Work out the finished part from the listing and answer in its coordinate system (mm). Coordinates: 2 decimals unless noted, no trailing zeros. Order: outer loops, then holes, each group sorted by start corner. A loop starts at its lowest first (then second) coordinate and runs counter-clockwise, first axis right, second up.
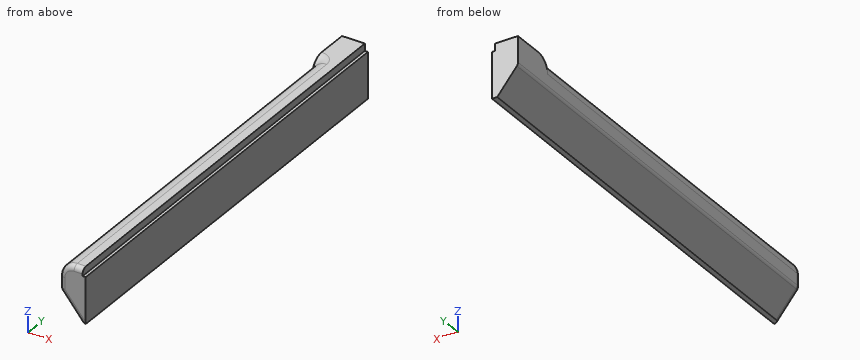
```python
from build123d import *

# Parameters (mm, degrees)
F1_DEPTH = 430
F3_W     = 14
F3_H     = 3.9684094482
F5_DEPTH = 385.0010001
F6_R     = 5


with BuildPart() as f1:
    # F0 (on Front) → F1 (new body)
    with BuildSketch(Plane.XZ):
        with BuildLine():
            Line((-3.0895532303, -0.0301503569), (-25.4895532303, -0.0301503569))
            Line((-25.4895532303, -0.0301503569), (-25.4895532303, -25.2490202056))
            ThreePointArc((-25.4895532303, -25.2490202056), (-25.1996290257, -26.9268718085), (-24.3634788298, -28.4101434948))
            Line((-24.3634788298, -28.4101434948), (-5.0895532303, -52.0301503569))
            Line((-5.0895532303, -52.0301503569), (-0.0895532303, -52.0301503569))
            Line((-0.0895532303, -52.0301503569), (-0.0895532303, -7.0301503569))
            Line((-0.0895532303, -7.0301503569), (-3.0895532303, -7.0301503569))
            Line((-3.0895532303, -7.0301503569), (-3.0895532303, -0.0301503569))
        make_face()
    extrude(amount=-F1_DEPTH)

    # F3 (on offset) → F4 (revolve, cut)
    with BuildSketch(Plane(origin=(0, 385, 0), x_dir=(-1, 0, 0), z_dir=(0, 1, 0))):
        with BuildLine():
            Line((25.4895532303, -14.0301503569), (25.4895532303, -0.0301503569))
            Line((25.4895532303, -0.0301503569), (11.4895532303, -0.0301503569))
            ThreePointArc((11.4895532303, -0.0301503569), (21.3890481669, -4.1306554203), (25.4895532303, -14.0301503569))
        make_face()
        with Locations((18.4895532303, 1.9540543671)):
            Rectangle(F3_W, F3_H)
    revolve(axis=Axis((-25.4895532303, 385, -5.0459456329), (0, 0, -1)), mode=Mode.SUBTRACT)

    # F3 (on offset) → F5 (cut, through all)
    with BuildSketch(Plane(origin=(0, 385, 0), x_dir=(-1, 0, 0), z_dir=(0, 1, 0))):
        with BuildLine():
            Line((25.4895532303, -14.0301503569), (25.4895532303, -0.0301503569))
            Line((25.4895532303, -0.0301503569), (11.4895532303, -0.0301503569))
            ThreePointArc((11.4895532303, -0.0301503569), (21.3890481669, -4.1306554203), (25.4895532303, -14.0301503569))
        make_face()
        with Locations((18.4895532303, 1.9540543671)):
            Rectangle(F3_W, F3_H)
    extrude(amount=-F5_DEPTH, mode=Mode.SUBTRACT)

    # F6
    f6_edges = [f1.edges().sort_by_distance(p)[0] for p in [
        (-7.289553, 0, -0.03015),
    ]]
    fillet(f6_edges, radius=F6_R)


solid = f1.part
```
1. Consider probe 1 along X at (y, z) = (399.5, -26); probe 2 along Y at (x, z) = (-18, -30); probe 3 along Y at (x, z) = (-5.25, -4.5). Determine where each line is inside the solid, lowest interval first.
2. The part is cut by section A-A (y = 211.5). Determine the outline of the cut face in (x, z), plus the area to 3 significant figures.
3. Flat-ended cylindrical pins translate along their axes: pin 1 (5 mm diameter, centred on x = -15.5, y = 182.5, fed in from -Z); pin 2 (8 mm diameter, centred on y = 156, z = -34.5, fed in from -X); pin 3 (1 mm diameter, centred on x = -15, y = 373, fed in from +Z). Find the tip coordinate at first contact, or state that the pin passes through.
Worked out:
1. probe 1: x = -25.43 to -0.09
1. probe 2: y = 0.12 to 430
1. probe 3: y = 0.03 to 430
2. outline: (-25.49, -25.25) arc R5 ccw to (-24.36, -28.41) - (-5.09, -52.03) - (-0.09, -52.03) - (-0.09, -7.03) - (-3.09, -7.03) - (-3.09, -0.03) - (-11.49, -0.03) arc R14 ccw to (-25.49, -14.03) - close
2. area: 1,000 mm2
3. pin 1: stops at z = -42.34
3. pin 2: stops at x = -22.66
3. pin 3: stops at z = -0.36
